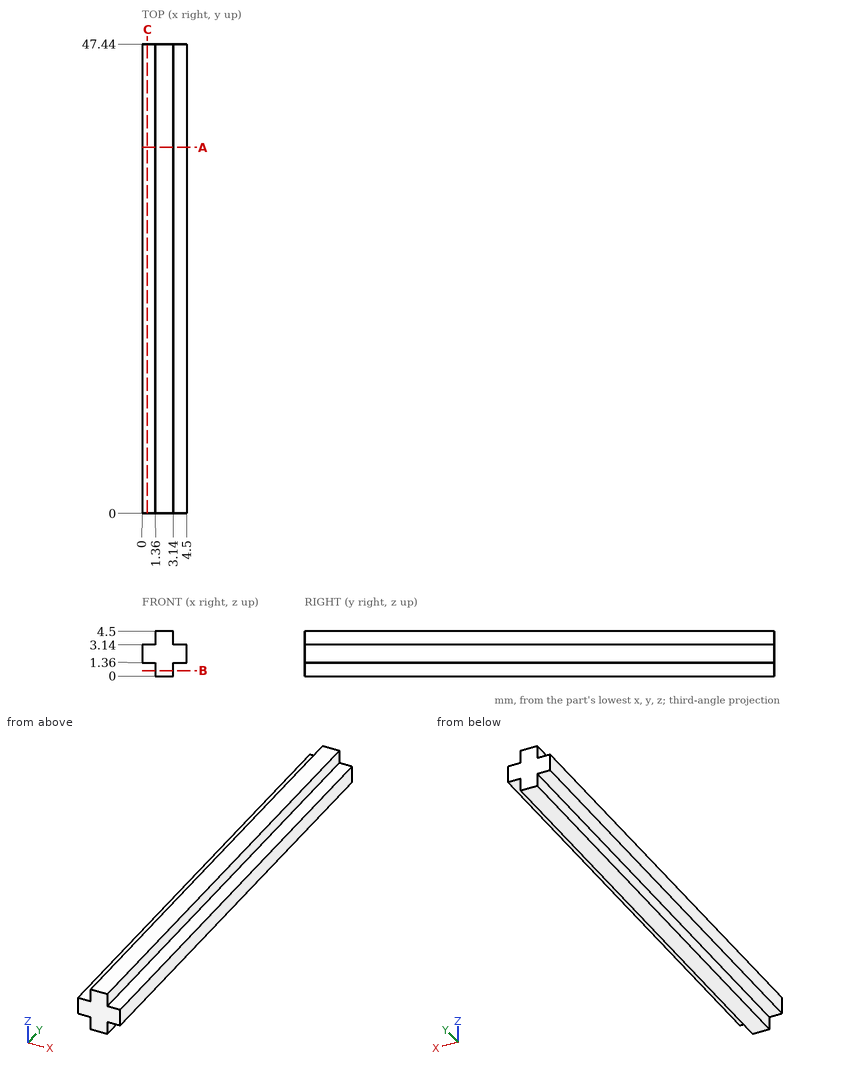
The drawing under review shows one solid part. Ordinate dimensions are in mm from its lowest x, y, z. Give positions to 0.01 mm unless a question says otherwise; leave off trailing zeros. Write each loop counter-clockwise with the first axis right and the second up, starting at its lowest first coordinate (ties: lowest second). Pieces come first, ordered by that corner, then holes. Notation, with made-up numbers: (-18.75, 60.25) -> (36.25, 60.25) arc R23 ccw to (36.25, 99.25) -> close; hole circle Ø1 at (1.5, 87). An arc over 180 degrees is marked (long way). Put each result on its own line as item: value.
(1) We need section B-B, the plane z = 0.55. Give the boundary of the cut face in (x, y).
Results are:
outline: (1.36, 0) -> (3.14, 0) -> (3.14, 47.44) -> (1.36, 47.44) -> close
(2) We need section A-A, the plane y = 37. Give the boundary of the cut face in (x, z), and give its area (3 significant figures).
Results are:
outline: (0, 1.36) -> (1.36, 1.36) -> (1.36, 0) -> (3.14, 0) -> (3.14, 1.36) -> (4.5, 1.36) -> (4.5, 3.14) -> (3.14, 3.14) -> (3.14, 4.5) -> (1.36, 4.5) -> (1.36, 3.14) -> (0, 3.14) -> close
area: 12.9 mm²
(3) To check wall thickness, follow probe 1 along Z at (x, y) = (1.25, 36). State the ranges of the line that lie inside material, in increasing order. Write a range as from..to.
Results are:
probe 1: 1.36..3.14
(4) For pin 1 Ø0.7 at (x, y) = (0.5, 18.5) entering from +Z; pin 2 Ø1.1 at (x, y) = (4, 32) entering from -Z; pin 3 Ø1.5 at (y, z) = (22, 0.5) entering from +X, all flat-tipped, find the tip position at first contact; note any pin that passes through.
Results are:
pin 1: z = 3.14
pin 2: z = 1.36
pin 3: x = 3.14
(5) We need section C-C, the plane x = 0.55. Give the boundary of the cut face in (y, z), and give its area (3 significant figures).
Results are:
outline: (0, 1.36) -> (47.44, 1.36) -> (47.44, 3.14) -> (0, 3.14) -> close
area: 84.4 mm²
